For this review, take the finished solid that the model builds, in its own axes (mm). Face numbers are marked on the shaded views. A direction names the side the tool comes from. Coordinates: 2 decimals unless noted, no trailing zeros. Loops run counter-clockwise (first coordinate to the right, second up) from the corner with the lowest first, then second, coordinate; pieces in that order, holes last. Notation, with made-up numbers: (82, 48.25) -> (134, 48.25) arc R12 cw to (134, 71.25) -> close; hole circle Ø7 at (37.5, -38.75). An arc over 180 degrees is marked (long way). Use a Markdown table: item, result.
from build123d import *

# Parameters (mm, degrees)
BASE_FLANGE1_DEPTH           = 0.81
EDGE_FLANGE1_STRIP_W         = 4.7132
EDGE_FLANGE1_STRIP_H         = 0.81
EDGE_FLANGE1_STRIP_CUT_DEPTH = 20
EDGE_FLANGE1_DEPTH           = 20
CUT_EXTRUDE1_REACH           = 38.455
SKETCH9_R                    = 2
CUT_EXTRUDE2_REACH           = 38.455
SKETCH10_R                   = 2


# Sheet-metal steps are written as plain solids
with BuildPart() as part:
    # Sketch1 → Base-Flange1 (new body)
    with BuildSketch(Plane.XY):
        with BuildLine():
            Line((0, 0), (20, 0))
            Line((20, 0), (20, 10))
            ThreePointArc((20, 10), (10, 20), (0, 10))
            Line((0, 10), (0, 0))
        make_face()
    extrude(amount=-BASE_FLANGE1_DEPTH)

    # Edge-Flange1 strip (across the edge) → Edge-Flange1 strip cut (cut)
    with BuildSketch(Plane.YZ):
        with Locations((-1.62, -0.405)):
            Rectangle(EDGE_FLANGE1_STRIP_W, EDGE_FLANGE1_STRIP_H)
    extrude(amount=EDGE_FLANGE1_STRIP_CUT_DEPTH, mode=Mode.SUBTRACT)

    # Edge-Flange1 section (across the edge) → Edge-Flange1 (add)
    with BuildSketch(Plane.YZ):
        with BuildLine():
            Line((-0.81, 0.7366), (-0.81, 23))
            Line((-0.81, 23), (0, 23))
            Line((0, 23), (0, 0.7366))
            ThreePointArc((0, 0.7366), (0.215745145, 0.215745145), (0.7366, 0))
            Line((0.7366, 0), (0.7366, -0.81))
            ThreePointArc((0.7366, -0.81), (-0.357011348, -0.357011348), (-0.81, 0.7366))
        make_face()
    extrude(amount=EDGE_FLANGE1_DEPTH)

    # Sketch9 → Cut-Extrude1 (cut, up to next)
    with BuildSketch(Plane.XY, mode=Mode.PRIVATE) as cut_extrude1_sk1:
        with Locations((10, 10)):
            Circle(SKETCH9_R)
    cut_extrude1_tool1 = extrude(cut_extrude1_sk1.sketch, amount=-CUT_EXTRUDE1_REACH, mode=Mode.PRIVATE) & part.part
    add(cut_extrude1_tool1.solids().sort_by_distance((10, 10, 0))[0], mode=Mode.SUBTRACT)

    # Sketch10 → Cut-Extrude2 (cut, up to next)
    with BuildSketch(Plane(origin=(0, 0, 0), x_dir=(1, 0, 0), z_dir=(0, 1, 0)), mode=Mode.PRIVATE) as cut_extrude2_sk1:
        with Locations(Location((10, -11.87, 0), (0, 0, 270))):
            Circle(SKETCH10_R)
    cut_extrude2_tool1 = extrude(cut_extrude2_sk1.sketch, amount=-CUT_EXTRUDE2_REACH, mode=Mode.PRIVATE) & part.part
    add(cut_extrude2_tool1.solids().sort_by_distance((10, 0, 11.87))[0], mode=Mode.SUBTRACT)


solid = part.part
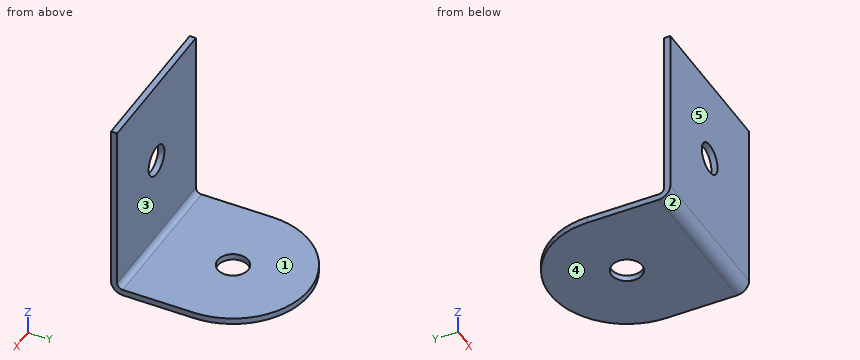
(1) Mouldability with a two-part tool opening along Y and no side actions: class the marked faces 3, 4 and 5 as pulls with the +Y half, pulls with the -Y half, needs draft (parallel to the pull), parting line crosses it, or undercut.
Found:
| item | result |
|---|---|
| face 3 | pulls with the +Y half |
| face 4 | needs draft |
| face 5 | pulls with the -Y half |
(2) Take a section at B-B on z = 12.75. Write out the cut boundary in (x, y), plus the area to 3 significant figures.
Found:
| item | result |
|---|---|
| outline | (0, -0.81) -> (8.2, -0.81) -> (8.2, 0) -> (0, 0) -> close; (11.8, -0.81) -> (20, -0.81) -> (20, 0) -> (11.8, 0) -> close |
| area | 13.3 mm^2 |
(3) For the marked faces 1 and 2, list the 3-axis set-ups (+Z, -Z, +X, -X, +Y, -Y) from which the entire face can be reached by the end or side of a thin tool; tool diameter is ignored.
Found:
| item | result |
|---|---|
| face 1 | +Z, +X, -X, +Y |
| face 2 | -Z, +X, -X, -Y |
(4) Take a section at A-A on x = 10. Write out the cut boundary in (y, z).
Found:
| item | result |
|---|---|
| outline | (-0.81, 0.74) arc R1.55 ccw to (0.74, -0.81) -> (8, -0.81) -> (8, 0) -> (0.74, 0) arc R0.74 cw to (0, 0.74) -> (0, 9.87) -> (-0.81, 9.87) -> close; (-0.81, 13.87) -> (0, 13.87) -> (0, 23) -> (-0.81, 23) -> close; (12, -0.81) -> (20, -0.81) -> (20, 0) -> (12, 0) -> close |
(5) Take a section at D-D on x = 14. Write out the cut boundary in (y, z).
Found:
| item | result |
|---|---|
| outline | (-0.81, 0.74) arc R1.55 ccw to (0.74, -0.81) -> (19.17, -0.81) -> (19.17, 0) -> (0.74, 0) arc R0.74 cw to (0, 0.74) -> (0, 23) -> (-0.81, 23) -> close |
(6) For line 1 along X through (y, z) = (-0.25, 11.87); line 2 along Y through (x, z) = (19.25, 8.75), list the stretches that pass through material, from the lowest coordinate up.
Found:
| item | result |
|---|---|
| line 1 | x = 0 to 8, 12 to 20 |
| line 2 | y = -0.81 to 0 |
(7) For pin 1 Ø6 at (x, z) = (3, 13.5) entering from +Y; pin 2 Ø6 at (x, y) = (7.5, 11) entering from +Z, all flat-tipped, find the tip position at first contact; note any pin that passes through.
Found:
| item | result |
|---|---|
| pin 1 | stops at y = 0 |
| pin 2 | stops at z = 0 |
(8) Take a section at C-C on y = 7.5. Write out the cut boundary in (x, z), plus the area to 3 significant figures.
Found:
| item | result |
|---|---|
| outline | (0, -0.81) -> (20, -0.81) -> (20, 0) -> (0, 0) -> close |
| area | 16.2 mm^2 |
